```python
from build123d import *

# Parameters (mm, degrees)
SKETCH_1_W      = 170
SKETCH_1_H      = 150
SKETCH_1_R      = 1.5
SKETCH_1_R_2    = 1.9
EXTRUDE_1_DEPTH = 5
FILLET_1_R      = 5
FILLET_2_R      = 40


with BuildPart() as part:
    # 草图1 → 凸台-拉伸1 (new body)
    with BuildSketch(Plane(origin=(0, 0, 0), x_dir=(1, 0, 0), z_dir=(0, 1, 0))):
        with Locations((-4, 0)):
            Rectangle(SKETCH_1_W, SKETCH_1_H)
        with Locations((75, 18)):
            Circle(SKETCH_1_R, mode=Mode.SUBTRACT)
        with Locations((18, 18)):
            Circle(SKETCH_1_R, mode=Mode.SUBTRACT)
        with Locations((-83.25, 17.75)):
            Circle(SKETCH_1_R_2, mode=Mode.SUBTRACT)
        with Locations((-9.58, -59.5)):
            Circle(SKETCH_1_R, mode=Mode.SUBTRACT)
        with Locations((-83, 34)):
            Circle(SKETCH_1_R_2, mode=Mode.SUBTRACT)
        with Locations((-83, 69)):
            Circle(SKETCH_1_R_2, mode=Mode.SUBTRACT)
        with Locations((-33, 34)):
            Circle(SKETCH_1_R_2, mode=Mode.SUBTRACT)
        with Locations((-33, 69)):
            Circle(SKETCH_1_R_2, mode=Mode.SUBTRACT)
        with Locations((-12, 34)):
            Circle(SKETCH_1_R_2, mode=Mode.SUBTRACT)
        with Locations((-12, 69)):
            Circle(SKETCH_1_R_2, mode=Mode.SUBTRACT)
        with Locations((38, 69)):
            Circle(SKETCH_1_R_2, mode=Mode.SUBTRACT)
        with Locations((38, 34)):
            Circle(SKETCH_1_R_2, mode=Mode.SUBTRACT)
        with Locations((-38.75, 17.75)):
            Circle(SKETCH_1_R_2, mode=Mode.SUBTRACT)
        with Locations((-18, 18)):
            Circle(SKETCH_1_R, mode=Mode.SUBTRACT)
        with Locations((39, 18)):
            Circle(SKETCH_1_R, mode=Mode.SUBTRACT)
        with Locations((75, -18)):
            Circle(SKETCH_1_R, mode=Mode.SUBTRACT)
        with Locations((39, -18)):
            Circle(SKETCH_1_R, mode=Mode.SUBTRACT)
        with Locations((18, -18)):
            Circle(SKETCH_1_R, mode=Mode.SUBTRACT)
        with Locations((-18, -18)):
            Circle(SKETCH_1_R, mode=Mode.SUBTRACT)
        with Locations((-83, -69)):
            Circle(SKETCH_1_R_2, mode=Mode.SUBTRACT)
        with Locations((-33, -69)):
            Circle(SKETCH_1_R_2, mode=Mode.SUBTRACT)
        with Locations((-33, -34)):
            Circle(SKETCH_1_R_2, mode=Mode.SUBTRACT)
        with Locations((-83, -34)):
            Circle(SKETCH_1_R_2, mode=Mode.SUBTRACT)
        with Locations((-38.75, -17.75)):
            Circle(SKETCH_1_R_2, mode=Mode.SUBTRACT)
        with Locations((-83.25, -17.75)):
            Circle(SKETCH_1_R_2, mode=Mode.SUBTRACT)
        with Locations((40.58, -59.5)):
            Circle(SKETCH_1_R, mode=Mode.SUBTRACT)
        with Locations((40.58, -32.5)):
            Circle(SKETCH_1_R, mode=Mode.SUBTRACT)
        with Locations((-9.58, -32.5)):
            Circle(SKETCH_1_R, mode=Mode.SUBTRACT)
    extrude(amount=EXTRUDE_1_DEPTH)

    # 圆角1
    fillet_1_edges = [part.edges().sort_by_distance(p)[0] for p in [
        (-89, 2.5, -75),
        (-89, 2.5, 75),
    ]]
    fillet(fillet_1_edges, radius=FILLET_1_R)

    # 圆角2
    fillet_2_edges = [part.edges().sort_by_distance(p)[0] for p in [
        (81, 2.5, -75),
        (81, 2.5, 75),
    ]]
    fillet(fillet_2_edges, radius=FILLET_2_R)


solid = part.part
```
Geometry check sheet. Reference: the model listing, model coordinates, mm. Coordinates: 2 decimals unless noted, no trailing zeros. Order: outer loops, then holes, each group sorted by start corner. A loop starts at its lowest first (then second) coordinate and runs counter-clockwise, first axis right, second up. Notation, with made-up numbers: M 42,20.25 L 58,20.25 A18 cw 58,55.25 Z; hole C 19.25,21 d1. An arc over 180 degrees is marked long. One line per question, with ' | ' between items. Start each with the question number.
Item 1: Cross-section at B-B on y = 1.35. State how many separate pieces and enclosed holes the cut face has, then the cut area to 3 significant figures.
Item 2: Gauge pin test, flat end, axial feed: pin 1 (1 mm diameter, centred on y = 1.5, z = -44, fed in from +X). Record the tip position at first contact, or that the pin passes through.
Item 3: Draft check along X on faces 1 (the cylindrical face through (-88, 3, -73)), 2 (the flat face through (-22, 2, -75)), 3 (the cylindrical face through (39.755, 2.465, -33.272)). Enter one of: pulls with the +X half, pulls with the -X half, needs draft (parallel to the pull), parting line crosses it, or undercut.
Item 4: Material ranges on L1, parallel to Z at x = 18, y = 0.3; L2, parallel to Z at x = -9.58, y = 1.35; L3, parallel to X at y = 2.25, z = -34, recorded low to high. Write a range as [from, to].
Item 5: Cross-section at A-A on x = -38.75. Enter the section's corners in (y, z).
Findings:
1) separate pieces: 1 | enclosed holes: 28 | area: 24,500 mm²
2) pin 1: stops at x = 80.09
3) face 1: pulls with the -X half | face 2: needs draft | face 3: undercut
4) L1: z = [-75, -19.5], [-16.5, 16.5], [19.5, 75] | L2: z = [-75, 31], [34, 58], [61, 75] | L3: x = [-89, -84.9], [-81.1, -34.9], [-31.1, -13.9], [-10.1, 36.1], [39.9, 81]
5) outline: M 0,-75 L 5,-75 L 5,-19.65 L 0,-19.65 Z; M 0,-15.85 L 5,-15.85 L 5,15.85 L 0,15.85 Z; M 0,19.65 L 5,19.65 L 5,75 L 0,75 Z
